```python
from build123d import *

# Parameters (mm, degrees)
F0_W     = 370
F0_H     = 10
F1_DEPTH = 1500


with BuildPart() as f1:
    # F0 (on Top) → F1 (new body)
    with BuildSketch(Plane.XY):
        Polygon((185, -227), (195, -227), (195, 227), (185, 227), (185, 217), (185, 5), (185, -5), (185, -217), align=None)
        Rectangle(F0_W, F0_H)
        Polygon((-185, -217), (-185, -5), (-185, 5), (-185, 217), (-185, 227), (-195, 227), (-195, -227), (-108.172141, -227), (-108.172141, -217), align=None)
    extrude(amount=F1_DEPTH)


solid = f1.part
```
Can you work these out from the model? Positions are in its coordinate system, mm. A direction names the side the tool comes from. Round coordinates to 2 decimals unless told otherwise and drop trailing zeros. Loops run counter-clockwise (first coordinate to the right, second up) from the corner with the lowest first, then second, coordinate; pieces in that order, holes last. Notation, with made-up numbers: M 62,-28.5 L 108,-28.5 A24 cw 108,-16.5 Z; hole C -10,89 d10. An arc over 180 degrees is marked long. Answer as a JSON object with one key per item and string values. Group by question number.
Q1. Will these pins go through, and if not, where does the flat tip stop? pin 1 (4 mm diameter, centred on x = -49.5, z = 925, fed in from -Y); pin 2 (3 mm diameter, centred on x = 148.5, z = 760.5, fed in from +Y).
Q2. Imagine slicing it at C-C, the plane x = 6.5. Please give me the cut outline in (y, z).
Q3. On a 3-axis mill with a long thin cutter (end or side, diameter ignored), from which of +Z, -Z, +X, -X, +Y, -Y can I reach the whole of each face in a straight line? I mean faces 1 (the flat face through (-146, -217, 740)), 2 (the flat face through (185, 118, 740)), 3 (the flat face through (-152, -227, 740)). Say none if no direction works.
Q4. Please list where these lines run through material, in increasing order: L1, parallel to X at y = -159, z = 464; L2, parallel to Y at x = -172, z = 879; L3, parallel to Y at x = -88, z = 819.
Q5. Imagine slicing it at A-A, the plane y = 182. Please give me the cut outline in (x, z).
Q6. Imagine slicing it at B-B, the plane z = 1329. Please give me the cut outline in (x, y), then the cut area to 3 significant figures.
Q7. We'd pull the mould along X, two halves only. Please class faces 4 (the flat face through (-15, 1, 0)), 5 (the flat face through (-195, 3, 740)), 6 (the flat face through (185, -114, 740)), 7 (the flat face through (195, -3, 740)): +X half, -X half, draft (parallel to the pull), parting line (faces both ways), or undercut.
Findings:
{
 "1": {"pin 1": "stops at y = -5", "pin 2": "stops at y = 5"},
 "2": {"outline": "M -5,0 L 5,0 L 5,1500 L -5,1500 Z"},
 "3": {"face 1": "+Z, -Z", "face 2": "+Z, -Z, +Y", "face 3": "+Z, -Z, +X, -X, -Y"},
 "4": {"L1": "x = -195 to -185, 185 to 195", "L2": "y = -227 to -217, -5 to 5", "L3": "y = -5 to 5"},
 "5": {"outline": "M -195,0 L -185,0 L -185,1500 L -195,1500 Z; M 185,0 L 195,0 L 195,1500 L 185,1500 Z"},
 "6": {"outline": "M -195,-227 L -108.17,-227 L -108.17,-217 L -185,-217 L -185,-5 L 185,-5 L 185,-227 L 195,-227 L 195,227 L 185,227 L 185,5 L -185,5 L -185,227 L -195,227 Z", "area": "13,500 mm2"},
 "7": {"face 4": "draft", "face 5": "-X half", "face 6": "undercut", "face 7": "+X half"}
}
